```python
from build123d import *

# Parameters (mm, degrees)
SKETCH1_R               = 72.39
SKETCH1_R_2             = 62.39
BOSS_EXTRUDE1_DEPTH     = 75
CUT_EXTRUDE1_DEPTH      = 73.39
CUT_EXTRUDE1_DEPTH_BACK = 73.39
CHAMFER1_SIZE           = 5
CHAMFER1_SIZE2          = 18.660254038


with BuildPart() as part:
    # Sketch1 → Boss-Extrude1 (new body)
    with BuildSketch(Plane(origin=(0, 0, 0), x_dir=(1, 0, 0), z_dir=(0, 1, 0))):
        Circle(SKETCH1_R)
        Circle(SKETCH1_R_2, mode=Mode.SUBTRACT)
    extrude(amount=BOSS_EXTRUDE1_DEPTH)

    # Sketch2 → Cut-Extrude1 (cut, two sides)
    with BuildSketch(Plane.XY) as cut_extrude1_sk:
        with BuildLine():
            Line((5, 28.839745962), (5, 23.839745962))
            Line((5, 23.839745962), (-5, 23.839745962))
            Line((-5, 23.839745962), (-5, 28.839745962))
            ThreePointArc((-5, 28.839745962), (-10, 37.5), (-5, 46.160254038))
            Line((-5, 46.160254038), (-5, 51.160254038))
            Line((-5, 51.160254038), (5, 51.160254038))
            Line((5, 51.160254038), (5, 46.160254038))
            ThreePointArc((5, 46.160254038), (10, 37.5), (5, 28.839745962))
        make_face()
    extrude(amount=CUT_EXTRUDE1_DEPTH, mode=Mode.SUBTRACT)
    extrude(cut_extrude1_sk.sketch, amount=-CUT_EXTRUDE1_DEPTH_BACK, mode=Mode.SUBTRACT)

    # Chamfer1
    chamfer1_edges = [part.edges().sort_by_distance(p)[0] for p in [
        (-62.39, 75, 0),
    ]]
    chamfer1_side = [part.faces().sort_by_distance(p)[0] for p in [
        (-70.342501604, 75, 0),
    ]]
    chamfer(chamfer1_edges, length=CHAMFER1_SIZE, length2=CHAMFER1_SIZE2, reference=chamfer1_side[0])


solid = part.part
```
CAD build for the part. Positions are in the model's coordinates, mm. A direction names the side the tool comes from. Give positions to 0.01 mm unless a question says otherwise; leave off trailing zeros. Write each loop counter-clockwise with the first axis right and the second up, starting at its lowest first coordinate (ties: lowest second). Pieces come first, ordered by that corner, then holes. Notation, with made-up numbers: M 55.5,13.5 L 96.5,13.5 A23 ccw 96.5,41.5 Z; hole C 20.25,-8 d8. An arc over 180 degrees is marked long. Return JSON: item names as keys, results as strings. Group by question number.
(1) Band-saw the part on C-C (y = 40). Give the cut face in (x, z).
(2) Mould opens along X. For faces 1 (the face through (-5, 49, 67)), 2 (the face through (48, 75, 48)) say: pulls with the +X half, pulls with the -X half, needs draft (parallel to the pull), parting line crosses it, or undercut.
(3) Flat gauge pins, fed straight in: pin 1 Ø5.5 at (y, z) = (47.5, -68.5) entering from +X; pin 2 Ø12 at (y, z) = (56.5, -40.5) entering from -X; pin 3 Ø8 at (x, y) = (30, 19.5) entering from +Z; pin 4 Ø5 at (x, z) = (-2.5, 65.5) entering from +Y. Where does each tip first touch, or does it go through?
(4) 3-axis set-ups, long thin cutter, end or side, ignore diameter. For faces 3 (the face through (0, 23.84, -67)), 4 (the face through (32, 0, -54)): which of +Z, -Z, +X, -X, +Y, -Y reach the whole face in a straight line?
(5) Drill centre lines: L1, parallel to X at y = 15.5, z = 0; L2, parallel to Z at x = 59.5, y = 68. Where is each one in solid material? Low to high. Write a range as [from, to].
(6) Band-saw the part on A-A (z = 0). Give the cut face in (x, y), and give its area (3 significant figures).
(7) Band-saw the part on D-D (y = 13). Give the cut face in (x, z).
(8) Band-saw the part on B-B (x = 0). Give the cut face in (y, z), and give its area (3 significant figures).
Entries:
{
 "1": {"outline": "M -9.68,-71.74 L -9.68,-61.63 A62.39 cw -9.68,61.63 L -9.68,71.74 A72.39 ccw Z; M 9.68,-71.74 A72.39 ccw 9.68,71.74 L 9.68,61.63 A62.39 cw 9.68,-61.63 Z"},
 "2": {"face 1": "undercut", "face 2": "needs draft"},
 "3": {"pin 1": "stops at x = 30.29", "pin 2": "stops at x = -63.64", "pin 3": "stops at z = 67.56", "pin 4": "stops at y = 75"},
 "4": {"face 3": "+Z, -Z", "face 4": "+Z, -Z, +X, -X, -Y"},
 "5": {"L1": "x = [-72.39, -62.39], [62.39, 72.39]", "L2": "z = [-41.23, -27.42], [27.42, 41.23]"},
 "6": {"outline": "M -72.39,0 L -62.39,0 L -62.39,56.34 L -67.39,75 L -72.39,75 Z; M 62.39,0 L 72.39,0 L 72.39,75 L 67.39,75 L 62.39,56.34 Z", "area": "1,410 mm^2"},
 "7": {"outline": "C 0,0 d144.78; hole C 0,0 d124.78"},
 "8": {"outline": "M 0,-72.39 L 23.84,-72.39 L 23.84,-62.39 L 0,-62.39 Z; M 0,62.39 L 23.84,62.39 L 23.84,72.39 L 0,72.39 Z; M 51.16,-72.39 L 75,-72.39 L 75,-67.39 L 56.34,-62.39 L 51.16,-62.39 Z; M 51.16,62.39 L 56.34,62.39 L 75,67.39 L 75,72.39 L 51.16,72.39 Z", "area": "860 mm^2"}
}
